Geometry: see drawing. Coordinates: mm, zero at the bounding-box minimum. A direction names the side the tool comes from. Coordinates: 2 decimals unless noted, no trailing zeros. Write each loop counter-clockwise with the first axis right and the second up, starting at its lowest first coordinate (ties: lowest second). Pieces come first, ordered by that corner, then holes. Notation, with made-up numbers: (0, 82) - (18, 82) arc R16 ccw to (18, 107) - close; hole circle Ø7 at (20, 77). An arc over 180 degrees is marked (long way). One line per question, with ' | ' between items. Start each with the question number.
Q1. Contact query for flat-ended pins moving along their axis: P1, Ø1.5, axis at x = 3, y = 11.5, coming from the +Z side; P2, Ø1.5, axis at y = 6, z = 24, coming from the -X side; P3, Ø8, axis at y = 9.5, z = 25.5, coming from the +X side. Output: stop coordinate, or through.
Q2. Access query for the marked faces 1 and 2. Directions: +Z, -Z, +X, -X, +Y, -Y. A direction counts if a zero-diameter tool reaches every point of the face in a straight line with its end or side. Return the directions, or none.
Q3. Line query: line 1 (Z direction, x = 15.5, y = 14.25); line 2 (Z direction, x = 9, y = 5.25); line 3 (X direction, y = 13, z = 17.5). Output: solid intervals per line, ascending.
Q4. Cut plane A-A, the plane z = 49. Return loops of the section in (x, y), plus the area to 3 significant figures.
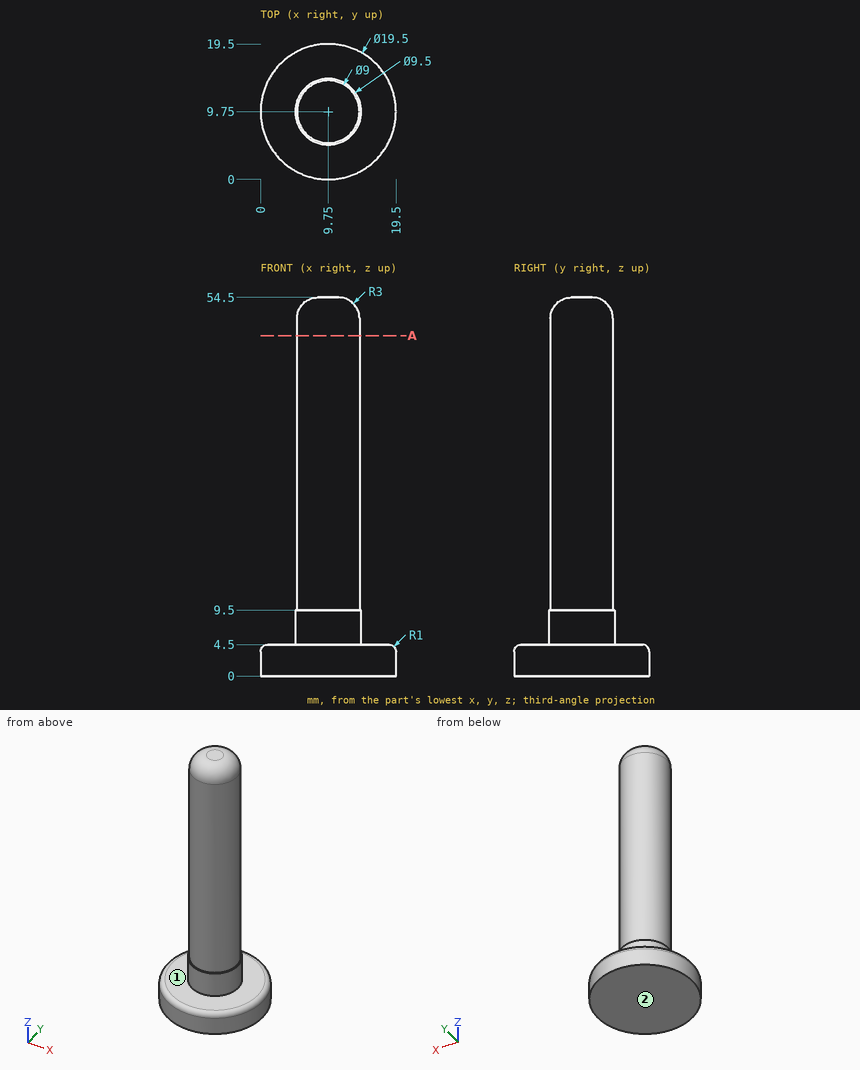
Reply:
1) P1: stops at z = 4.5 | P2: stops at x = 6.4 | P3: stops at x = 14.25
2) face 1: +Z | face 2: -Z, +X, -X, +Y, -Y
3) line 1: z = 0 to 4.5 | line 2: z = 0 to 9.5 | line 3: x = 6.64 to 12.86
4) outline: circle Ø9 at (9.75, 9.75) | area: 63.6 mm^2
